```python
from build123d import *

# Parameters (mm, degrees)
SKIZZE1_W                       = 173
SKIZZE1_H                       = 158
AUFSATZ_LINEAR_AUSTRAGEN1_DEPTH = 12
VERRUNDUNG1_R                   = 10
SKIZZE2_R                       = 74
AUFSATZ_LINEAR_AUSTRAGEN2_DEPTH = 132
SKIZZE3_R                       = 58
AUFSATZ_LINEAR_AUSTRAGEN3_DEPTH = 14.5
SKIZZE4_R                       = 6.75
SCHNITT_LINEAR_AUSTRAGEN1_DEPTH = 12
VERRUNDUNG2_R                   = 3
SKALIEREN1_SCALE                = 2


with BuildPart() as part:
    # Skizze1 → Aufsatz-Linear austragen1 (new body)
    with BuildSketch(Plane.XY):
        with Locations((86.5, 79)):
            Rectangle(SKIZZE1_W, SKIZZE1_H)
    extrude(amount=AUFSATZ_LINEAR_AUSTRAGEN1_DEPTH)

    # Verrundung1
    verrundung1_edges = [part.edges().sort_by_distance(p)[0] for p in [
        (0, 158, 6),
        (173, 158, 6),
        (173, 0, 6),
        (0, 0, 6),
    ]]
    fillet(verrundung1_edges, radius=VERRUNDUNG1_R)

    # Skizze2 → Aufsatz-Linear austragen2 (add)
    with BuildSketch(Plane.XY.offset(12)):
        with Locations((79, 79)):
            Circle(SKIZZE2_R)
    extrude(amount=AUFSATZ_LINEAR_AUSTRAGEN2_DEPTH)

    # Skizze3 → Aufsatz-Linear austragen3 (add)
    with BuildSketch(Plane.XY.offset(144)):
        with Locations(Location((79, 79, 0), (0, 0, 180))):
            Circle(SKIZZE3_R)
    extrude(amount=AUFSATZ_LINEAR_AUSTRAGEN3_DEPTH)

    # Skizze4 → Schnitt-Linear austragen1 (cut)
    with BuildSketch(Plane(origin=(0, 0, 0), x_dir=(-1, 0, 0), z_dir=(0, 0, -1))):
        with Locations((-163, 148)):
            Circle(SKIZZE4_R)
        with Locations((-10, 148)):
            Circle(SKIZZE4_R)
        with Locations((-10, 10)):
            Circle(SKIZZE4_R)
        with Locations((-163, 10)):
            Circle(SKIZZE4_R)
    extrude(amount=-SCHNITT_LINEAR_AUSTRAGEN1_DEPTH, mode=Mode.SUBTRACT)

    # Verrundung2
    verrundung2_edges = [part.edges().sort_by_distance(p)[0] for p in [
        (5, 79, 12),
    ]]
    fillet(verrundung2_edges, radius=VERRUNDUNG2_R)


with BuildPart() as part_1:
    # Skalieren1: scaled about (0, 0, 0)
    add(part.part.scale(SKALIEREN1_SCALE))


solid = part_1.part
```
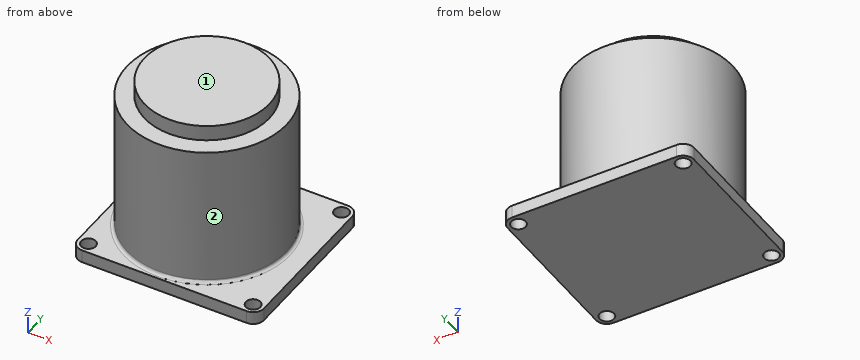
Input: part model. Units: mm. Frame: model coordinates. Face numbers are marked on the shaded views. A direction names the side the tool comes from. Give positions to 0.01 mm unless a question says otherwise; leave off trailing zeros. Order: outer loops, then holes, each group sorted by start corner. A loop starts at its lowest first (then second) coordinate and runs counter-clockwise, first axis right, second up. Notation, with made-up numbers: M 89.5,26.25 L 112.5,26.25 A10 ccw 112.5,43.25 Z; hole C 40.5,53 d10. An arc over 180 degrees is marked long. Return JSON: item names as keys, results as strings.
1) Access query for the marked faces 1 and 2. Directions: +Z, -Z, +X, -X, +Y, -Y. A direction counts if a zero-diameter tool reaches every point of the face in a straight line with its end or side. Return the directions, or none.
Taken from the geometry:
{"face 1": "+Z, +X, -X, +Y, -Y", "face 2": "+Z"}
2) Section query B-B on y = 158. Output: boundary loops of the cut face in (x, z).
Taken from the geometry:
{"outline": "M 0,0 L 346,0 L 346,24 L 312,24 A6 cw 306,30 L 306,288 L 274,288 L 274,317 L 42,317 L 42,288 L 10,288 L 10,30 A6 cw 4,24 L 0,24 Z"}
3) Contact query for flat-ended pins moving along their axis: pin 1 (21.5 mm diameter, centred on x = 326, y = 20, fed in from +Z); pin 2 (12 mm diameter, centred on x = 245.5, z = 73.5, fed in from -Y); pin 3 (12 mm diameter, centred on y = 58.5, z = 85.5, fed in from -X); pin 4 (5 mm diameter, centred on y = 65, z = 131.5, fed in from -X). Output: stop coordinate, or through.
Taken from the geometry:
{"pin 1": "passes through", "pin 2": "stops at y = 34.46", "pin 3": "stops at x = 43.28", "pin 4": "stops at x = 40.89"}
4) Section query C-C on z = 101. Output: boundary loops of the cut face in (x, y).
Taken from the geometry:
{"outline": "C 158,158 d296"}
5) Section query A-A on x = 158. Output: boundary loops of the cut face in (y, z).
Taken from the geometry:
{"outline": "M 0,0 L 316,0 L 316,24 L 312,24 A6 cw 306,30 L 306,288 L 274,288 L 274,317 L 42,317 L 42,288 L 10,288 L 10,30 A6 cw 4,24 L 0,24 Z"}
6) Line query: L1, parallel to Y at x = 20, z = 10.5; L2, parallel to Z at x = 84, y = 253.5; L3, parallel to X at y = 160.5, z = 221.5. Output: solid intervals per line, ascending. Write a range as [from, to].
Taken from the geometry:
{"L1": "y = [0, 6.5], [33.5, 282.5], [309.5, 316]", "L2": "z = [0, 288]", "L3": "x = [10.02, 305.98]"}
